Verification items for the finished model (mm, model axes). A direction names the side the tool comes from. Coordinates: 2 decimals unless noted, no trailing zeros. Order: outer loops, then holes, each group sorted by start corner. A loop starts at its lowest first (then second) coordinate and runs counter-clockwise, first axis right, second up. Notation, with made-up numbers: M -12.75,2.25 L 13.25,2.25 A21 ccw 13.25,32.25 Z; hole C -16.75,67.25 d8. An arc over 180 degrees is marked long. Write item = value, one per line.
```python
from build123d import *

# Parameters (mm, degrees)
SKETCH1_R           = 2.413
SKETCH1_R_2         = 0.75
BOSS_EXTRUDE1_DEPTH = 2


with BuildPart() as part:
    # Sketch1 → Boss-Extrude1 (new, symmetric)
    with BuildSketch(Plane(origin=(0, 0, 0), x_dir=(0, 0, -1), z_dir=(1, 0, 0))):
        with BuildLine():
            Line((-4.180666535, 6.35), (0, 6.35))
            ThreePointArc((0, 6.35), (4.490128061, 4.490128061), (6.35, 0))
            Line((6.35, 0), (6.35, -43.06614877))
            Line((6.35, -43.06614877), (-6.35, -43.06614877))
            Line((-6.35, -43.06614877), (-6.35, -11.43))
            ThreePointArc((-6.35, -11.43), (-7.837897552, -7.837897552), (-11.43, -6.35))
            Line((-11.43, -6.35), (-43.06614877, -6.35))
            Line((-43.06614877, -6.35), (-43.06614877, 6.35))
            Line((-43.06614877, 6.35), (-39.60826893, 18.780106665))
            Line((-39.60826893, 18.780106665), (-13.871980247, 11.620635214))
            ThreePointArc((-13.871980247, 11.620635214), (-13.07637114, 11.325756262), (-12.340940682, 10.902566601))
            Line((-12.340940682, 10.902566601), (-7.073190955, 7.253913018))
            ThreePointArc((-7.073190955, 7.253913018), (-5.695902182, 6.5812413), (-4.180666535, 6.35))
        make_face()
        Circle(SKETCH1_R, mode=Mode.SUBTRACT)
        with Locations((-5.1, -38.06614877)):
            Circle(SKETCH1_R_2, mode=Mode.SUBTRACT)
        with Locations((-2.954545455, -38.06614877)):
            Circle(SKETCH1_R_2, mode=Mode.SUBTRACT)
        with Locations((-0.809090909, -38.06614877)):
            Circle(SKETCH1_R_2, mode=Mode.SUBTRACT)
        with Locations((1.336363636, -38.06614877)):
            Circle(SKETCH1_R_2, mode=Mode.SUBTRACT)
        with Locations((3.481818182, -38.06614877)):
            Circle(SKETCH1_R_2, mode=Mode.SUBTRACT)
    extrude(amount=BOSS_EXTRUDE1_DEPTH, both=True)


solid = part.part
```
Item 1: Scan lines: L1, parallel to Y at x = 1.85, z = -2; L2, parallel to Z at x = 1, y = -16; L3, parallel to Y at x = -0.6, z = 2. Record each from-to range of solid material in increasing order. Write a range as from..to.
Report:
L1 = -43.07..-38.42, -37.72..-1.35, 1.35..6.03
L2 = -6.35..6.35
L3 = -43.07..-1.35, 1.35..6.35
Item 2: Sectioned sample at A-A, the plane z = 5.1. Enter the section's corners in (x, y).
Report:
outline = M -2,-43.07 L 2,-43.07 L 2,-38.82 L -2,-38.82 Z; M -2,-37.32 L 2,-37.32 L 2,6.43 L -2,6.43 Z
Item 3: Sectioned sample at C-C, the plane x = 1.1. Enter the section's corners in (y, z).
Report:
outline = M -43.07,-6.35 L 0,-6.35 A6.35 ccw 6.35,0 L 6.35,4.18 A5.08 cw 7.25,7.07 L 10.9,12.34 A5.08 ccw 11.62,13.87 L 18.78,39.61 L 6.35,43.07 L -6.35,43.07 L -6.35,11.43 A5.08 cw -11.43,6.35 L -43.07,6.35 Z; hole C -38.07,-3.48 d1.5; hole C -38.07,-1.34 d1.5; hole C -38.07,0.81 d1.5; hole C -38.07,2.95 d1.5; hole C -38.07,5.1 d1.5; hole C 0,0 d4.83
Item 4: Gauge pin test, flat end, axial feed: pin 1 (1 mm diameter, centred on x = -1, y = 2, fed in from -Z). Record the tip position at first contact, or that the pin passes through.
Report:
pin_1 = -6.17
Item 5: Sectioned sample at B-B, the plane y = -14. Enter the section's corners in (x, z).
Report:
outline = M -2,-6.35 L 2,-6.35 L 2,6.35 L -2,6.35 Z
Item 6: Sectioned sample at D-D, the plane z = 27.5. Enter the section's corners in (x, y).
Report:
outline = M -2,-6.35 L 2,-6.35 L 2,15.41 L -2,15.41 Z
Item 7: Release check for a two-part mould opening along Z. For faces 1 (the cylindrical face through (-0.03, -38.73, 0.46)), 2 (the cylindrical face through (0.03, 6.59, 5.72)), 3 (the flat face through (0, -27, 6.35)) record: pulls with the +Z half, pulls with the -Z half, needs draft (parallel to the pull), parting line crosses it, or undercut.
Report:
face_1 = undercut
face_2 = pulls with the -Z half
face_3 = pulls with the +Z half
Item 8: Tool access check on faces 4 (the flat face through (0, 6.35, 2)), 5 (the flat face through (0, -6.35, 27)), 6 (the cylindrical face through (-0.028, -1.468, 1.915)). Record the directions out of +Z, -Z, +X, -X, +Y, -Y that give a thin tool (end or side, any length) a straight path to the whole face; none if there is none.
Report:
face_4 = -Z, +X, -X, +Y
face_5 = +Z, +X, -X, -Y
face_6 = +X, -X
